Answer from the drawing. Dimensions are ordinates in mm from the lowest x, y and z of the part. Round coordinates to 2 decimals unless told otherwise and drop trailing zeros. Loops run counter-clockwise (first coordinate to the right, second up) from the corner with the lowest first, then second, coordinate; pieces in that order, holes last. Notation, with made-up numbers: (29.25, 38) -> (77.25, 38) arc R26 cw to (77.25, 53) -> close; hole circle Ø11 at (-8.75, 27.25). An arc over 180 degrees is marked (long way). Use CSV: the item, a comma, the result in double quotes. Start each with the question number.
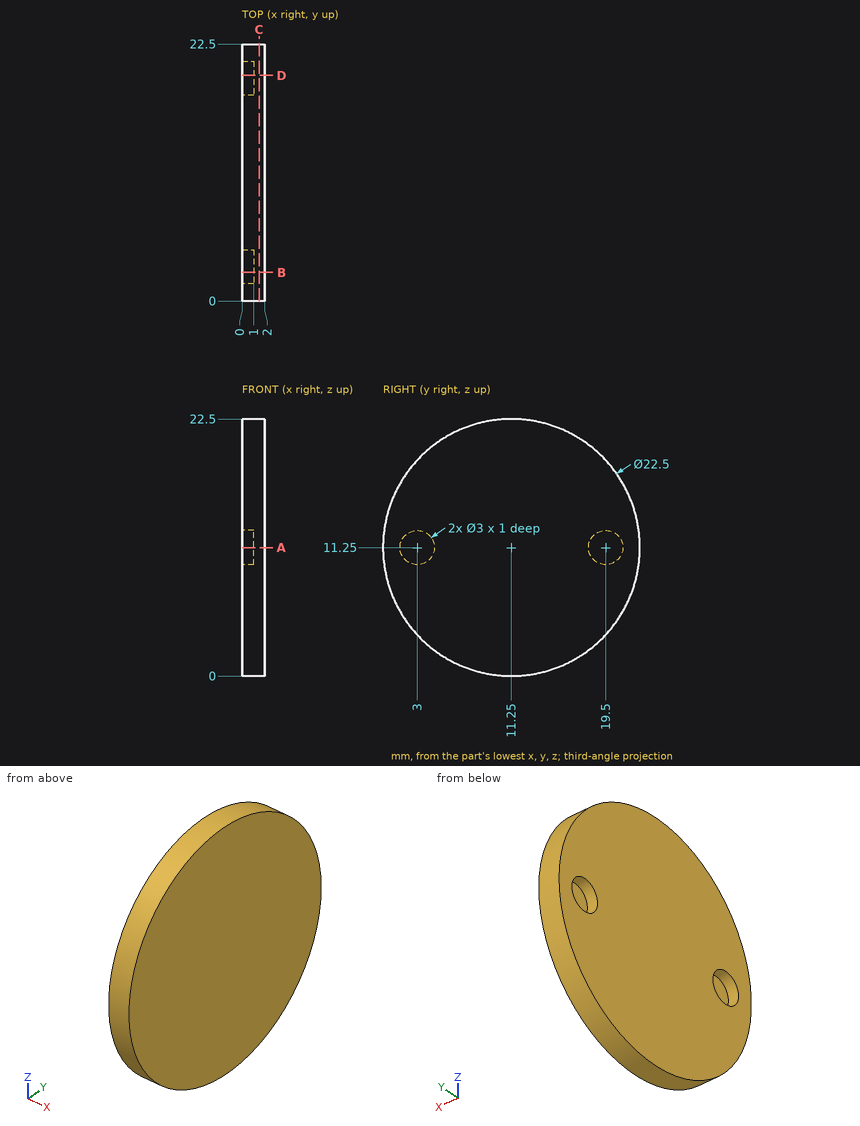
Q1. Section D-D, the plane y = 19.75 is taken. Write down the section's boundary in (x, z).
Q2. Each of these flat-tipped pins is pushed along its axis until it touches: pin 1 (1 mm diameter, centred on x = 0.5, z = 19, fed in from -Y); pin 2 (0.9 mm diameter, centred on y = 3.5, z = 12, fed in from -X). Where does it stop, or does it pass through?
Q3. Straight lines are drawn through the part: line 1 (Z direction, x = 0.3, y = 19.25); line 2 (Z direction, x = 0.5, y = 3); line 3 (Z direction, x = 1.7, y = 6). For each, find the intervals that lie inside material, in ascending order. Write a range as from..to.
Q4. Section B-B, the plane y = 2.5 is taken. Write down the section's boundary in (x, z), and give its area (3 significant figures).
Q5. Section A-A, the plane z = 11.25 is taken. Write down the section's boundary in (x, y).
Q6. Section C-C, the plane x = 1.5 is taken. Write down the section's boundary in (y, z), and give its area (3 significant figures).
Report:
1,outline,"(0, 3.88) -> (2, 3.88) -> (2, 18.62) -> (0, 18.62) -> (0, 12.73) -> (1, 12.73) -> (1, 9.77) -> (0, 9.77) -> close"
2,pin 1,"stops at y = 2.65"
2,pin 2,"stops at x = 1"
3,line 1,"z = 3.34..9.77, 12.73..19.16"
3,line 2,"z = 3.6..9.75, 12.75..18.9"
3,line 3,"z = 1.3..21.2"
4,outline,"(0, 4.18) -> (2, 4.18) -> (2, 18.32) -> (0, 18.32) -> (0, 12.66) -> (1, 12.66) -> (1, 9.84) -> (0, 9.84) -> close"
4,area,"25.5 mm²"
5,outline,"(0, 0) -> (2, 0) -> (2, 22.5) -> (0, 22.5) -> (0, 21) -> (1, 21) -> (1, 18) -> (0, 18) -> (0, 4.5) -> (1, 4.5) -> (1, 1.5) -> (0, 1.5) -> close"
6,outline,"circle Ø22.5 at (11.25, 11.25)"
6,area,"398 mm²"
